The model under review builds one solid part; all positions refer to its coordinate system, in mm. A direction names the side the tool comes from. Coordinates: 2 decimals unless noted, no trailing zeros. Write each loop counter-clockwise with the first axis right and the second up, starting at its lowest first coordinate (ties: lowest second). Pieces come first, ordered by that corner, then holes. Notation, with made-up numbers: (37, 20) - (71, 20) arc R7 cw to (71, 31) - close; hole circle Ø3 at (26.25, -16.75). An arc over 180 degrees is marked (long way). Answer as CSV lines item,"result". Start each with the question number.
Autodesk Inventor part; units mm, degrees
ref_plane "YZ Plane" through (0, 0, 0) normal (1, 0, 0) x (0, 1, 0)
ref_plane "XZ Plane" through (0, 0, 0) normal (0, 1, 0) x (-1, 0, 0)
ref_plane "XY Plane" through (0, 0, 0) normal (0, 0, 1) x (1, 0, 0)
sketch "Sketch4" plane through (0, 0, 0) normal (0, 0, 1) x (1, 0, 0)
  line L0 (-10.5, 0) -> (10.5, 0)
  line L1 (0, -3.3) -> (0, 19.8)
  line L2 (-7.5, 0) -> (7.5, 0)
  line L3 (7.5, 0) -> (7.5, 16.5)
  line L4 (7.5, 16.5) -> (-7.5, 16.5)
  line L5 (-7.5, 16.5) -> (-7.5, 0)
  circle A0 centre (0, 10) radius 2.5
  point P0 (0, 0)
  dimension "d0" = 7.5
  dimension "d1" = 7.5
  dimension "d2" = 16.5
  dimension "d3" = 5
  dimension "d4" = 6.5
extrude "Extrusion1" add sketch "Sketch4" against normal blind 15.9 contours L5 L4 L1 A0 L0 | L1 A0 L4 L3 L0
fillet "Fillet1" radius 7.5 2 edges at (7.5, 16.5, -7.95) (-7.5, 16.5, -7.95)
sketch "Sketch13" plane through (7.5, 9, 0) normal (1, 0, 0) x (0, 0, -1)
  line L0 (0, -12.3) -> (0, 10.8)
  line L1 (19.08, -9) -> (-3.18, -9)
  line L2 (0, -9) -> (0, 0)
  line L3 (0, 7.5) -> (15.9, 7.5)
  line L4 (0, -9) -> (2.7, -9)
  line L5 (2.7, -9) -> (2.7, 7.5)
  line L6 (2.7, 7.5) -> (0, 7.5)
  line L7 (0, 7.5) -> (0, -9)
  line L8 (15.9, -9) -> (15.9, 0)
  line L9 (15.9, -9) -> (13.2, -9)
  line L10 (13.2, -9) -> (13.2, 7.5)
  line L11 (13.2, 7.5) -> (15.9, 7.5)
  line L12 (15.9, 7.5) -> (15.9, -9)
  line L13 (6.6, -9) -> (9.3, -9)
  line L14 (9.3, -9) -> (9.3, 7.5)
  line L15 (9.3, 7.5) -> (6.6, 7.5)
  line L16 (6.6, 7.5) -> (6.6, -9)
  dimension "d47" = 2.7
  dimension "d48" = 2.7
  dimension "d49" = 2.7
  dimension "d50" = 15.9
  dimension "d51" = 3.9
  dimension "d52" = 3.9
extrude "Extrusion8" cut sketch "Sketch13" against normal through all contours L5 L3 L16 L1 | L14 L3 L10 L1
sketch "Sketch14" plane through (-7.5, 0, -6.6) normal (0, -1, 0) x (1, 0, 0)
  line L0 (0, 6.6) -> (15, 6.6)
  line L1 (15, -9.3) -> (0, -9.3)
  line L2 (15, 6.6) -> (0, 6.6)
  line L3 (0, 6.6) -> (0, -9.3)
  line L4 (0, -9.3) -> (15, -9.3)
  line L5 (15, -9.3) -> (15, 6.6)
  point P0 (7.5, 6.6)
extrude "Extrusion9" add sketch "Sketch14" along normal blind 4
properties part number "mountGeneric"
(1) The part is to be moulded in two halves that separate along X. For faces 3 (the flat face through (0, 6, 0)), 4 (the cylindrical face through (-5.361, 14.245, -7.969)), 5 (the cylindrical face through (-0.54, 7.56, -14.53)), say which applies: released by +X, released by -X, zero draft, split by the parting line, or undercut.
(2) Add section C-C on x = -0.75. Give the boundary of the cut face in (y, z), then the cut area to 3 significant figures.
(3) Wall thickness on line 1 (Z direction, x = 1.75, y = 15); line 2 (Y direction, x = 0, z = -15.1); line 3 (Y direction, x = 1, z = -8): over which ranges is each line inside the solid? List them lowest first.
(4) Add section B-B on y = 6.25. Give the boundary of the cut face in (x, z).
(5) For pin 1 (8 mm diameter, centred on x = -4.5, z = -13, fed in from +Y); pin 2 (1.2 mm diameter, centred on x = 3.5, z = -11.5, fed in from +Y); pin 3 (8 mm diameter, centred on y = 13.5, z = -13.5, fed in from -X); pin 4 (4 mm diameter, centred on x = 0, y = 10, fed in from -Z), all flat-tipped, find the tip position at first contact; note any pin that passes through.
(6) Add section D-D on y = 10. Give the boundary of the cut face in (x, z).
(7) For faces 1 (the flat face through (0, 0, -5)), 2 (the cylindrical face through (5.245, 14.361, -1.369)), list the 3-axis set-ups (+Z, -Z, +X, -X, +Y, -Y) from which the entire face can be reached by the end or side of a thin tool; tool diameter is ignored.
Reported:
1,face 3,"zero draft"
1,face 4,"released by -X"
1,face 5,"undercut"
2,outline,"(-4, -15.9) - (7.62, -15.9) - (7.62, -13.2) - (0, -13.2) - (0, -9.3) - (7.62, -9.3) - (7.62, -6.6) - (0, -6.6) - (0, -2.7) - (7.62, -2.7) - (7.62, 0) - (-4, 0) - close; (12.38, -15.9) - (16.46, -15.9) - (16.46, -13.2) - (12.38, -13.2) - close; (12.38, -9.3) - (16.46, -9.3) - (16.46, -6.6) - (12.38, -6.6) - close; (12.38, -2.7) - (16.46, -2.7) - (16.46, 0) - (12.38, 0) - close"
2,area,"158 mm²"
3,line 1,"-15.9 to -13.2, -9.3 to -6.6, -2.7 to 0"
3,line 2,"-4 to 7.5, 12.5 to 16.5"
3,line 3,"-4 to 7.71, 12.29 to 16.43"
4,outline,"(-7.5, -15.9) - (7.5, -15.9) - (7.5, -13.2) - (-7.5, -13.2) - close; (-7.5, -9.3) - (7.5, -9.3) - (7.5, -6.6) - (-7.5, -6.6) - close; (-7.5, -2.7) - (7.5, -2.7) - (7.5, 0) - (-7.5, 0) - close"
5,pin 1,"y = 16.48"
5,pin 2,"y = 0"
5,pin 3,"x = -7.48"
5,pin 4,"through"
6,outline,"(-7.43, -15.9) - (-2.5, -15.9) - (-2.5, -13.2) - (-7.43, -13.2) - close; (-7.43, -9.3) - (-2.5, -9.3) - (-2.5, -6.6) - (-7.43, -6.6) - close; (-7.43, -2.7) - (-2.5, -2.7) - (-2.5, 0) - (-7.43, 0) - close; (2.5, -15.9) - (7.43, -15.9) - (7.43, -13.2) - (2.5, -13.2) - close; (2.5, -9.3) - (7.43, -9.3) - (7.43, -6.6) - (2.5, -6.6) - close; (2.5, -2.7) - (7.43, -2.7) - (7.43, 0) - (2.5, 0) - close"
7,face 1,"+X, -X, +Y"
7,face 2,"+Z, -Z, +X, +Y"
